Read the model definition and answer for the solid it produces. Units are mm, in the model's axes. A direction names the side the tool comes from. Coordinates: 2 decimals unless noted, no trailing zeros. Write each loop counter-clockwise with the first axis right and the second up, starting at its lowest first coordinate (ties: lowest second). Pieces come first, ordered by that corner, then holes. Notation, with made-up numbers: (-26.5, 71) -> (-5.5, 71) arc R22 ccw to (-5.5, 92) -> close; hole circle Ø10 at (-14, 40.5). An arc over 180 degrees is marked (long way). Write item = value, one per line. Start each with the question number.
1) For a pull along Y with two mould halves and no side action, classify faces 1 (the face through (0, -4, -3)), 2 (the face through (-7.644, 4.565, -9.496)), 3 (the face through (-6, 0, 27)), 4 (the face through (7.616, -4.515, -9.06)) as released by +Y, released by -Y, zero draft, split by the parting line, or undercut.
2) Section A-A (z = 15) is taken. Determine the outline of the cut face in (x, y).
3) Flat-ended cylindrical pins translate along their axes: pin 1 Ø5 at (x, z) = (7, 47) entering from +Y; pin 2 Ø6 at (x, z) = (-1, 10) entering from +Y; pin 3 Ø1.7 at (x, y) = (0, 4) entering from -Z. Find the tip coordinate at first contact, or state that the pin passes through.
4) Find the intervals of material crossed by line 1 along Y through (x, z) = (0, 41.5); line 2 along Y through (x, z) = (0, 68); line 3 along Z through (x, y) = (8.5, 0.5), in increasing order. Write a range as from..to.
5) A tool of negligible diameter and unlimited length cuts with its end or side. For faces 5 (the face through (-1.5, 0.07, 69.63)), 6 (the face through (0, -4, -2)), 7 (the face through (7.615, 4.512, -9.943)), from which of +Z, -Z, +X, -X, +Y, -Y can it reach the whole face along a straight path? Write none if from no direction.
from build123d import *

# Parameters (mm, degrees)
F0_R          = 6
F0_R_2        = 5
F1_DEPTH      = 62
F1_DEPTH_BACK = 9
F6_DEPTH      = 1
F8_R          = 5
F9_DEPTH      = 1
F10_R         = 1
F11_R         = 0.2
F12_R         = 0.2


# Not quite as in the source:
# - a feature names something its author has since deleted; it is built from what else it names


with BuildPart() as f1:
    # F0 (on Top) → F1 (new body, two sides)
    with BuildSketch(Plane.XY) as f1_sk:
        Circle(F0_R)
        Circle(F0_R_2, mode=Mode.SUBTRACT)
    extrude(amount=F1_DEPTH)
    extrude(f1_sk.sketch, amount=-F1_DEPTH_BACK)

    # F2 (on Front) → F3 (revolve)
    with BuildSketch(Plane.XZ):
        with BuildLine():
            Line((6, 62), (4.6430466171, 62.5427813535))
            ThreePointArc((4.6430466171, 62.5427813535), (2.3596638473, 64.3820207615), (1.5, 67.1851648075))
            Line((1.5, 67.1851648075), (1.5, 72))
            Line((1.5, 72), (0.5, 72))
            Line((0.5, 72), (0.5, 63.8000000012))
            Line((0.5, 63.8000000012), (5, 62))
            Line((5, 62), (6, 62))
        make_face()
    revolve(axis=Axis((0, 0, 62.4439572394), (0, 0, 1)))

    # F5 (on offset) → F6 (join)
    with BuildSketch(Plane.XY.offset(-2)):
        with BuildLine():
            ThreePointArc((-3.5707142143, -3.5), (0, -5), (3.5707142143, -3.5))
            Line((3.5707142143, -3.5), (-3.5707142143, -3.5))
        make_face()
        with BuildLine():
            Line((-3.5707142143, 3.5), (3.5707142143, 3.5))
            ThreePointArc((3.5707142143, 3.5), (0, 5), (-3.5707142143, 3.5))
        make_face()
    extrude(amount=-F6_DEPTH)

    # F8 (on offset) → F9 (join)
    with BuildSketch(Plane(origin=(0, 0, -9), x_dir=(1, 0, 0), z_dir=(0, 0, -1))):
        Polygon((11, 2.7135847191), (4.4980677776, 6.3), (-4.4980677776, 6.3), (-11, 2.7135847191), (-11, -2.7135847191), (-4.4980677776, -6.3), (4.4980677776, -6.3), (11, -2.7135847191), align=None)
        Circle(F8_R, mode=Mode.SUBTRACT)
    extrude(amount=F9_DEPTH)

    # F10
    f10_edges = [f1.edges().sort_by_distance(p)[0] for p in [
        (11, -2.713585, -9.5),
        (4.498068, -6.3, -9.5),
        (11, 2.713585, -9.5),
        (-4.498068, -6.3, -9.5),
        (4.498068, 6.3, -9.5),
        (-11, -2.713585, -9.5),
        (-4.498068, 6.3, -9.5),
        (-11, 2.713585, -9.5),
    ]]
    fillet(f10_edges, radius=F10_R)

    # F11
    f11_edges = [f1.edges().sort_by_distance(p)[0] for p in [
        (-7.603269, -4.587195, -10),
        (-4.489932, -6.268408, -10),
        (0, -6.3, -10),
        (-11, 0, -10),
        (-10.861101, -2.631572, -10),
        (-10.861101, 2.631572, -10),
        (-7.603269, 4.587195, -10),
        (-4.489932, 6.268408, -10),
        (0, 6.3, -10),
        (4.489932, 6.268408, -10),
        (7.603269, 4.587195, -10),
        (7.603269, -4.587195, -10),
        (4.489932, -6.268408, -10),
        (10.861101, -2.631572, -10),
        (11, 0, -10),
        (10.861101, 2.631572, -10),
    ]]
    fillet(f11_edges, radius=F11_R)

    # F12
    f12_edges = [f1.edges().sort_by_distance(p)[0] for p in [
        (10.861101, -2.631572, -9),
        (11, 0, -9),
        (10.861101, 2.631572, -9),
        (7.603269, 4.587195, -9),
        (4.489932, 6.268408, -9),
        (0, 6.3, -9),
        (-4.489932, 6.268408, -9),
        (-10.861101, 2.631572, -9),
        (-7.603269, 4.587195, -9),
        (7.603269, -4.587195, -9),
        (0, -6.3, -9),
        (-11, 0, -9),
        (-10.861101, -2.631572, -9),
        (-4.489932, -6.268408, -9),
        (4.489932, -6.268408, -9),
        (-7.603269, -4.587195, -9),
    ]]
    fillet(f12_edges, radius=F12_R)


solid = f1.part
Answer key:
q1.face_1 = undercut
q1.face_2 = released by +Y
q1.face_3 = split by the parting line
q1.face_4 = released by -Y
q2.outline = circle Ø12 at (0, 0); hole circle Ø10 at (0, 0)
q3.pin_1 = 3.97
q3.pin_2 = 6
q3.pin_3 = -3
q4.line_1 = -6..-5, 5..6
q4.line_2 = -1.5..-0.5, 0.5..1.5
q4.line_3 = -10..-9
q5.face_5 = +Z
q5.face_6 = none
q5.face_7 = -Z, +X, +Y
